```python
from build123d import *

# Parameters (mm, degrees)
F2_R      = 1
F3_DEPTH  = 25
F2_R_2    = 1.9
F3_FACE_R = 1
F4_DEPTH  = 2
F5_SIZE   = 0.3
F7_DEPTH  = 1.3


with BuildPart() as f3:
    # F2 (on Top) → F3 (new body)
    with BuildSketch(Plane.XY):
        Circle(F2_R)
    extrude(amount=-F3_DEPTH)

    # F2 (on Top) + F3_face (on face) → F4 (join)
    with BuildSketch(Plane.XY):
        Circle(F2_R_2)
        Circle(F2_R, mode=Mode.SUBTRACT)
    with BuildSketch(Plane.XY):
        Circle(F3_FACE_R)
    extrude(amount=F4_DEPTH)

    # F5
    f5_edges = [f3.edges().sort_by_distance(p)[0] for p in [
        (-1, 0, -25),
        (-1.9, 0, 2),
    ]]
    chamfer(f5_edges, length=F5_SIZE)

    # F6 (on face) → F7 (cut)
    with BuildSketch(Plane.XY.offset(2)):
        Polygon((1, -0.5773502692), (1, 0.5773502692), (0, 1.1547005384), (-1, 0.5773502692), (-1, -0.5773502692), (0, -1.1547005384), align=None)
    extrude(amount=-F7_DEPTH, mode=Mode.SUBTRACT)


solid = f3.part
```
Geometry check sheet. Reference: the model listing, model coordinates, mm. A direction names the side the tool comes from. Give positions to 0.01 mm unless a question says otherwise; leave off trailing zeros. Loops run counter-clockwise (first coordinate to the right, second up) from the corner with the lowest first, then second, coordinate; pieces in that order, holes last. Notation, with made-up numbers: M 69,-31 L 94,-31 A22 ccw 94,1 Z; hole C 68,64 d2. An arc over 180 degrees is marked long. Answer as CSV lines item,"result".
Item 1: Cross-section at B-B on z = -11.25. Record the cut outline in (x, y).
Values:
outline,"C 0,0 d2"
Item 2: Depth check by flat-ended pin: P1, Ø2, axis at y = -0.5, z = -13, coming from the +X side; P2, Ø2, axis at y = -1, z = -1.5, coming from the -X side; P3, Ø0.6, axis at x = 0, y = 0, coming from the +Z side. Enter the tip coordinate at first touch or a pass-through.
Values:
P1,"stops at x = 1"
P2,"stops at x = -1"
P3,"stops at z = 0.7"
Item 3: Release check for a two-part mould opening along Y. For faces 4 (the flat face through (-1, 1, 2)), 5 (the cylindrical face through (0, -1, -12)), 6 (the flat face through (-1, 0, 1)) record: pulls with the +Y half, pulls with the -Y half, needs draft (parallel to the pull), parting line crosses it, or undercut.
Values:
face 4,"needs draft"
face 5,"parting line crosses it"
face 6,"undercut"
Item 4: Cross-section at A-A on y = 0. Record the cut outline in (x, z).
Values:
outline,"M -1.9,0 L -1,0 L -1,-24.7 L -0.7,-25 L 0.7,-25 L 1,-24.7 L 1,0 L 1.9,0 L 1.9,1.7 L 1.6,2 L 1,2 L 1,0.7 L -1,0.7 L -1,2 L -1.6,2 L -1.9,1.7 Z"
Item 5: Access from +Z, -Z, +X, -X, +Y, -Y to the whole of each face (thin tool, end or side, straight path). Record for faces 1 (the flat face through (0.51, 0.86, 1.36)), 2 (the flat face through (1, -1, 0)), 3 (the cylindrical face through (-1.9, 0.08, 0.84)).
Values:
face 1,"+Z"
face 2,"-Z"
face 3,"+Z, -Z"
Item 6: Material ranges on line 1 (Z direction, x = -0.2, y = -1.3); line 2 (Z direction, x = 0.5, y = 0.2); line 3 (Y direction, x = -0.1, z = -12.5), recorded low to high.
Values:
line 1,"z = 0 to 2"
line 2,"z = -25 to 0.7"
line 3,"y = -0.99 to 0.99"
